Model file for the job. Use its own axes, mm. A direction names the side the tool comes from. Give positions to 0.01 mm unless a question says otherwise; leave off trailing zeros. Loops run counter-clockwise (first coordinate to the right, second up) from the corner with the lowest first, then second, coordinate; pieces in that order, holes last. Notation, with made-up numbers: (-0.75, 84.25) - (29.25, 84.25) arc R22 ccw to (29.25, 112.25) - close; hole circle Ø10 at (-28, 50.25). An arc over 180 degrees is marked (long way). Answer as CSV lines item,"result". Start each with the question number.
Item 1: Saw through at D-D on x = 0. Give the cut face in (y, z), plus the area to 3 significant figures.
Item 2: Saw through at C-C on x = 8.75. Give the cut face in (y, z).
Item 3: Drill centre lines: L1, parallel to Z at x = -4.75, y = 3.45; L2, parallel to X at y = 3.9, z = 4; L3, parallel to Z at x = 5.75, y = 4.3. Where is each one in solid material? Low to high. Write a range as from..to.
Item 4: Tool access for faces 1 (the cylindrical face through (-3.92, 3.232, 6.742)), 2 (the cylindrical face through (2.42, 3.23, 8.77)), 3 (the flat face through (2, 3, 0)): list every direction of +Z, -Z, +X, -X, +Y, -Y with a clear straight run to the whole face (end or side of a thin tool).
Item 5: Pull direction X, two halves, no side cores. Call faces 4 (the flat face through (-2, 3, 0)), 5 (the flat face through (-6, 4.5, 0)), 6 (the cylindrical face through (-5.357, 0.986, 3.604)): pulls with the +X half, pulls with the -X half, needs draft (parallel to the pull), parting line crosses it, or undercut.
Item 6: Saw through at B-B on y = 1.45. Give the cut face in (x, z), plus the area to 3 significant figures.
Item 7: Saw through at A-A on z = 0. Give the cut face in (x, y), plus the area to 3 significant figures.
Item 8: Pin check, flat tips, straight feed: pin 1 (3 mm diameter, centred on x = 4.6, z = 4.6, fed in from -Y); pin 2 (1.2 mm diameter, centred on y = 3.5, z = -4, fed in from +X); pin 3 (2 mm diameter, centred on x = 4.6, z = -4.6, fed in from -Y); pin 4 (1.5 mm diameter, centred on y = 4, z = -4.5, fed in from -X). Stop position of each tip, or through.
from build123d import *

# Parameters (mm, degrees)
SKETCH_1_R      = 9.5
SKETCH_1_R_2    = 1.25
EXTRUDE_1_DEPTH = 2
SKETCH_2_R      = 2.25
EXTRUDE_2_DEPTH = 2.5


with BuildPart() as part:
    # 草图1 → 凸台-拉伸1 (new body)
    with BuildSketch(Plane(origin=(0, 0, 0), x_dir=(1, 0, 0), z_dir=(0, 1, 0))):
        with Locations(Location((0, 0, 0), (0, 0, 270))):
            Circle(SKETCH_1_R)
        with Locations(Location((4.596194078, 4.596194078, 0), (0, 0, 270))):
            Circle(SKETCH_1_R_2, mode=Mode.SUBTRACT)
        with Locations(Location((4.596194078, -4.596194078, 0), (0, 0, 270))):
            Circle(SKETCH_1_R_2, mode=Mode.SUBTRACT)
        with Locations(Location((-4.596194078, -4.596194078, 0), (0, 0, 270))):
            Circle(SKETCH_1_R_2, mode=Mode.SUBTRACT)
        with Locations(Location((-4.596194078, 4.596194078, 0), (0, 0, 270))):
            Circle(SKETCH_1_R_2, mode=Mode.SUBTRACT)
    extrude(amount=EXTRUDE_1_DEPTH)

    # 草图2 → 凸台-拉伸2 (add)
    # profile 1 of 2: a face of its own
    with BuildSketch(Plane(origin=(0, 2, 0), x_dir=(1, 0, 0), z_dir=(0, 1, 0))):
        with BuildLine():
            Line((-2, 7.95298686), (-2, -7.95298686))
            ThreePointArc((-2, -7.95298686), (-2.431203541, -8.775465181), (-3.352941176, -8.888632373))
            ThreePointArc((-3.352941176, -8.888632373), (-9.5, 0), (-3.352941176, 8.888632373))
            ThreePointArc((-3.352941176, 8.888632373), (-2.431203541, 8.775465181), (-2, 7.95298686))
        make_face()
        with Locations(Location((-4.596194078, 4.596194078, 0), (0, 0, 270))):
            Circle(SKETCH_2_R, mode=Mode.SUBTRACT)
        with Locations(Location((-4.596194078, -4.596194078, 0), (0, 0, 270))):
            Circle(SKETCH_2_R, mode=Mode.SUBTRACT)
    # profile 2 of 2: a face of its own
    with BuildSketch(Plane(origin=(0, 2, 0), x_dir=(1, 0, 0), z_dir=(0, 1, 0))):
        with BuildLine():
            Line((2, 7.95298686), (2, -7.95298686))
            ThreePointArc((2, -7.95298686), (2.431203541, -8.775465181), (3.352941176, -8.888632373))
            ThreePointArc((3.352941176, -8.888632373), (9.5, 0), (3.352941176, 8.888632373))
            ThreePointArc((3.352941176, 8.888632373), (2.431203541, 8.775465181), (2, 7.95298686))
        make_face()
        with Locations(Location((4.596194078, 4.596194078, 0), (0, 0, 270))):
            Circle(SKETCH_2_R, mode=Mode.SUBTRACT)
        with Locations(Location((4.596194078, -4.596194078, 0), (0, 0, 270))):
            Circle(SKETCH_2_R, mode=Mode.SUBTRACT)
    extrude(amount=EXTRUDE_2_DEPTH)


solid = part.part
Responses:
1,outline,"(0, -9.5) - (2, -9.5) - (2, 9.5) - (0, 9.5) - close"
1,area,"38.0 mm2"
2,outline,"(0, -3.7) - (4.5, -3.7) - (4.5, 3.7) - (0, 3.7) - close"
3,L1,"-8.23..-6.84, -2.35..2.35, 6.84..8.23"
3,L2,"-8.62..-6.77, -2.43..-2, 2..2.43, 6.77..8.62"
3,L3,"-7.56..-6.53, -2.66..2.66, 6.53..7.56"
4,face 1,"+Y"
4,face 2,"+Z, +Y"
4,face 3,"+Z, -Z, +Y"
5,face 4,"undercut"
5,face 5,"needs draft"
5,face 6,"undercut"
6,outline,"circle Ø19 at (0, 0); hole circle Ø2.5 at (-4.6, -4.6); hole circle Ø2.5 at (-4.6, 4.6); hole circle Ø2.5 at (4.6, -4.6); hole circle Ø2.5 at (4.6, 4.6)"
6,area,"264 mm2"
7,outline,"(-9.5, 0) - (9.5, 0) - (9.5, 4.5) - (2, 4.5) - (2, 2) - (-2, 2) - (-2, 4.5) - (-9.5, 4.5) - close"
7,area,"75.5 mm2"
8,pin 1,"y = 0"
8,pin 2,"x = 8.87"
8,pin 3,"through"
8,pin 4,"x = -8.73"
